Design review of the part built by this model. Coordinates are the model's own, in mm. Coordinates: 2 decimals unless noted, no trailing zeros. Loops run counter-clockwise (first coordinate to the right, second up) from the corner with the lowest first, then second, coordinate; pieces in that order, holes last. Notation, with made-up numbers: (-25.5, -21) -> (13.5, -21) arc R25 ccw to (13.5, -9) -> close; hole circle Ø10 at (22, 20). An arc over 180 degrees is marked (long way). Answer as a JSON object with one key per item and string values.
Autodesk Fusion 360 part; units mm, degrees
sketch "Sketch1" plane through (0, 0, 0) normal (0, 0, 1) x (1, 0, 0)
  line L0 (10, 0) -> (205, 0)
  line L1 (215, 10) -> (215, 60)
  line L2 (205, 70) -> (10, 70)
  line L3 (0, 60) -> (0, 10)
  arc A0 (10, 70) -> (0, 60) centre (10, 60) ccw
  arc A1 (0, 10) -> (10, 0) centre (10, 10) ccw
  arc A2 (215, 60) -> (205, 70) centre (205, 60) ccw
  arc A3 (205, 0) -> (215, 10) centre (205, 10) ccw
  line L4 (205, 70) -> (205, 0)
  circle A4 centre (205, 43.9323) radius 3.5
  circle A5 centre (205, 23.9323) radius 3.5
  line L5 (102.5, 70) -> (102.5, 0)
  line L6 (205, 43.9323) -> (102.5, 43.9323)
  line L7 (205, 23.9323) -> (102.5, 23.9323)
  circle A6 centre (102.5, 43.9323) radius 3.5
  circle A7 centre (102.5, 23.9323) radius 3.5
  line L8 (89, 60) -> (49, 60)
  line L9 (49, 60) -> (49, 10)
  line L10 (49, 10) -> (89, 10)
  line L11 (89, 10) -> (89, 60)
  line L12 (102.5, 35) -> (89, 35)
  line L13 (49, 52.5466) -> (19, 52.5466)
  line L14 (19, 52.5466) -> (19, 17.4534)
  line L15 (19, 17.4534) -> (49, 17.4534)
  line L16 (49, 17.4534) -> (49, 52.5466)
  line L17 (19, 35) -> (49, 35)
  line L18 (0, 0) -> (0, 24.1752)
  line L19 (0, 0) -> (-15.0158, 0)
  line L20 (89, 60) -> (19, 60)
  line L21 (19, 60) -> (19, 10)
  line L22 (19, 10) -> (89, 10)
  line L23 (89, 10) -> (89, 60)
  circle A8 centre (89, 60) radius 1.25
  circle A9 centre (89, 10) radius 1.25
  circle A10 centre (19, 10) radius 1.5
  circle A11 centre (19, 60) radius 1.25
  point P0 (215, 0)
  point P1 (215, 70)
  point P2 (0, 70)
  dimension "d1" = 215
  dimension "d2" = 70
  dimension "d3" = 10
  dimension "d4" = 10
  dimension "d5" = 10
  dimension "d6" = 10
  dimension "d7" = 10
  dimension "d8" = 7
  dimension "d9" = 7
  dimension "d10" = 20
  dimension "d11" = 102.5
  dimension "d12" = 7
  dimension "d13" = 7
  dimension "d14" = 40
  dimension "d15" = 50
  dimension "d16" = 90
  dimension "d17" = 13.5
  dimension "d18" = 30
  dimension "d19" = 90
  dimension "d20" = 2.5
  dimension "d21" = 2.5
  dimension "d22" = 3
  dimension "d23" = 2.5
extrude "Extrude1" add sketch "Sketch1" along normal blind 6 contours L8 L9 L10 L11 L16 L20 L22 L23 A8 A9 | L0 L2 L3 A0 A1 L5 A6 A7 L18 | L0 L4 A5 L5 L7 A7 | L1 A2 A3 L4 A4 A5 | L4 A4 A5 L5 L6 L7 A6 A7 | L2 L4 A4 L5 L6 A6 | L9 L15 L21 L22 A10 | L9 L13 L20 L21 A11 | L9 L14 L15 L16 L17 L21 | L9 L13 L14 L16 L17 L21
sketch "Sketch2" plane through (0, 0, 6) normal (0, 0, 1) x (-1, 0, 0)
  circle A0 centre (-19, -60) radius 1.25
  circle A1 centre (-102.5, -43.9323) radius 3.5
  circle A2 centre (-89, -60) radius 1.25
  circle A3 centre (-89, -10) radius 1.25
  circle A4 centre (-102.5, -23.9323) radius 3.5
  circle A5 centre (-19, -10) radius 1.5
  circle A6 centre (-205, -23.9323) radius 3.5
  circle A7 centre (-205, -43.9323) radius 3.5
  arc A8 (0, -10) -> (-10, 0) centre (-10, -10) ccw
  line L0 (-10, 0) -> (-205, 0)
  arc A9 (-205, 0) -> (-215, -10) centre (-205, -10) ccw
  line L1 (-215, -10) -> (-215, -60)
  arc A10 (-215, -60) -> (-205, -70) centre (-205, -60) ccw
  line L2 (-205, -70) -> (-10, -70)
  arc A11 (-10, -70) -> (0, -60) centre (-10, -60) ccw
  line L3 (0, -60) -> (0, -10)
  line L4 (-157.5, -70) -> (-157.5, 0)
  line L5 (-102.5, -43.9323) -> (-102.5, -23.9323)
  circle A12 centre (-157.5, -42.1823) radius 1.25
  circle A13 centre (-157.5, -25.6823) radius 1.25
  line L6 (-151.1278, -40.9323) -> (-166.7652, -40.9323)
  line L7 (-166.7652, -40.9323) -> (-166.7652, -26.9323)
  line L8 (-166.7652, -26.9323) -> (-151.1278, -26.9323)
  line L9 (-151.1278, -26.9323) -> (-151.1278, -40.9323)
  line L10 (-151.1278, -33.9323) -> (-102.5, -33.9323)
  dimension "d26" = 55
  dimension "d27" = 14
  dimension "d28" = 90
  dimension "d29" = 2.5
  dimension "d30" = 2.5
extrude "Extrude2" cut sketch "Sketch2" against normal blind 5 contours L4 A13 | L4 A13 | L4 A12 | L4 A12
sketch "Sketch3" plane through (0, 0, 6) normal (0, 0, 1) x (-1, 0, 0)
  circle A0 centre (-157.5, -42.1823) radius 1.25
  circle A1 centre (-157.5, -25.6823) radius 1.25
  circle A2 centre (-205, -43.9323) radius 3.5
  circle A3 centre (-19, -10) radius 1.5
  circle A4 centre (-89, -60) radius 1.25
  circle A5 centre (-89, -10) radius 1.25
  circle A6 centre (-102.5, -43.9323) radius 3.5
  circle A7 centre (-19, -60) radius 1.25
  circle A8 centre (-205, -23.9323) radius 3.5
  circle A9 centre (-102.5, -23.9323) radius 3.5
  arc A10 (0, -10) -> (-10, 0) centre (-10, -10) ccw
  line L0 (-10, 0) -> (-205, 0)
  arc A11 (-205, 0) -> (-215, -10) centre (-205, -10) ccw
  line L1 (-215, -10) -> (-215, -60)
  arc A12 (-215, -60) -> (-205, -70) centre (-205, -60) ccw
  line L2 (-205, -70) -> (-10, -70)
  arc A13 (-10, -70) -> (0, -60) centre (-10, -60) ccw
  line L3 (0, -60) -> (0, -10)
  line L4 (-6.5, -60) -> (-6.5, -10)
  circle A14 centre (-6.5, -35) radius 3.5
  line L5 (-10, -60) -> (-10, -10)
  line L6 (-6.5, -35) -> (0, -35)
  line L7 (-205, -70) -> (-205, 0)
  circle A15 centre (-205, -63) radius 3.5
  circle A16 centre (-205, -7) radius 3.5
  dimension "d33" = 7
  dimension "d36" = 7
  dimension "d37" = 7
  dimension "d38" = 7
  dimension "d39" = 7
extrude "Extrude3" cut sketch "Sketch3" against normal blind 7 contours L4 A14 L6 | L4 A14 L6 | L7 A15 | L7 A15 | L7 A16 | L7 A16 | L4 A14
extrude "Extrude4" cut 1 faces at (157.8221, 41.8565, 1) along direction (0, 0, -1) blind 5
extrude "Extrude5" cut 1 faces at (157.1946, 25.2747, 1) along direction (0, 0, -1) blind 5
1) Add section C-C, the plane z = 3.45. Count the separate pieces of the cut face and the enclosed holes in it, and give its area (3 significant figures).
Completed:
{"separate pieces": "1", "enclosed holes": "13", "area": "14,700 mm²"}
2) Wall thickness on probe 1 along Y at (x, z) = (89.5, 2.2); probe 2 along Y at (x, z) = (89, 2.5); probe 3 along Y at (x, z) = (205, 3.2): over which ranges is each line inside the solid? List them lowest first.
Completed:
{"probe 1": "0 to 8.85, 11.15 to 58.85, 61.15 to 70", "probe 2": "0 to 8.75, 11.25 to 58.75, 61.25 to 70", "probe 3": "0 to 3.5, 10.5 to 20.43, 27.43 to 40.43, 47.43 to 59.5, 66.5 to 70"}
3) The part is to be moulded in two halves that separate along X. For faces 1 (the cylindrical face through (212.15, 3.01, 2.96)), 2 (the cylindrical face through (201.66, 61.95, 3.04)), 3 (the cylindrical face through (2.85, 66.99, 2.96)), say which applies: pulls with the +X half, pulls with the -X half, needs draft (parallel to the pull), parting line crosses it, or undercut.
Completed:
{"face 1": "pulls with the +X half", "face 2": "undercut", "face 3": "pulls with the -X half"}
4) Add section A-A, the plane x = 102.5. Give the boundary of the cut face in (y, z).
Completed:
{"outline": "(0, 0) -> (20.43, 0) -> (20.43, 6) -> (0, 6) -> close; (27.43, 0) -> (40.43, 0) -> (40.43, 6) -> (27.43, 6) -> close; (47.43, 0) -> (70, 0) -> (70, 6) -> (47.43, 6) -> close"}
5) Add section B-B, the plane y = 35. Give the boundary of the cut face in (x, z).
Completed:
{"outline": "(0, 0) -> (3, 0) -> (3, 6) -> (0, 6) -> close; (10, 0) -> (215, 0) -> (215, 6) -> (10, 6) -> close"}
6) Clearance check with flat-ended pins moving along their axes: pin 1 Ø2.5 at (x, y) = (19, 10) entering from -Z; pin 2 Ø6 at (x, y) = (88, 20) entering from -Z. State where each tip first meets the part, or that it passes through.
Completed:
{"pin 1": "through", "pin 2": "z = 0"}
